Job drawing, mm, ordinate dimensions from the low corner. One solid piece. A direction names the side the tool comes from. Coordinates: 2 decimals unless noted, no trailing zeros. Loops run counter-clockwise (first coordinate to the right, second up) from the corner with the lowest first, then second, coordinate; pieces in that order, holes last. Notation, with made-up numbers: (30, 82) - (62, 82) arc R19 cw to (62, 93) - close; hole circle Ø9 at (81.25, -31.5). An arc over 180 degrees is marked (long way). Use a Markdown table: item, result. Add a question column.
1. Band-saw the part on A-A, the plane x = 11. Give the cut face in (y, z).
2. 3-axis set-ups, long thin cutter, end or side, ignore diameter. For the marked faces 4 and 5: which of +Z, -Z, +X, -X, +Y, -Y reach the whole face in a straight line?
3. Pull direction X, two halves, no side cores. Call the marked faces 1, 2 and 3: pulls with the +X half, pulls with the -X half, needs draft (parallel to the pull), parting line crosses it, or undercut.
4. Band-saw the part on D-D, the plane y = 19. Give the cut face in (x, z), plus the area to 3 significant figures.
5. Drop flat-ended pins along their axis: pin 1 (1.5 mm diameter, centred on x = 8.5, z = 2.5, fed in from +Y); pin 2 (1 mm diameter, centred on x = 3.5, z = 2, fed in from +Y); pin 3 (1.8 mm diameter, centred on x = 12.5, y = 12, fed in from +Z). Give the stop position or say it passes through.
6. Band-saw the part on C-C, the plane z = 0.5. Give the cut face in (x, y).
7. Wall check: probe 1 along Y at (x, z) = (11, 1.55); probe 2 along Y at (x, z) = (11, 2.2); probe 3 along X at (y, z) = (11.25, 0.5). Give the ranges that are in metal, low to high. Write a range as [from, to].
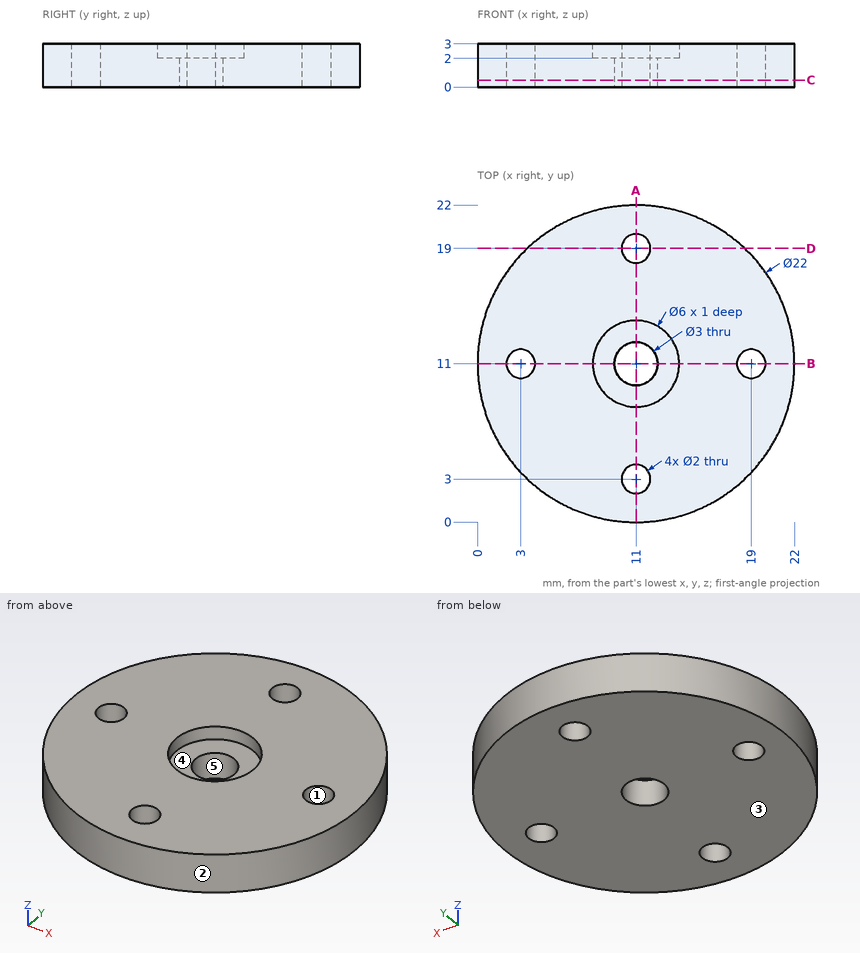
Geometry check:
| question | item | result |
|---|---|---|
| 1 | outline | (0, 0) - (2, 0) - (2, 3) - (0, 3) - close; (4, 0) - (9.5, 0) - (9.5, 2) - (8, 2) - (8, 3) - (4, 3) - close; (12.5, 0) - (18, 0) - (18, 3) - (14, 3) - (14, 2) - (12.5, 2) - close; (20, 0) - (22, 0) - (22, 3) - (20, 3) - close |
| 2 | face 4 | +Z |
| 2 | face 5 | +Z, -Z |
| 3 | face 1 | undercut |
| 3 | face 2 | parting line crosses it |
| 3 | face 3 | needs draft |
| 4 | outline | (3.45, 0) - (10, 0) - (10, 3) - (3.45, 3) - close; (12, 0) - (18.55, 0) - (18.55, 3) - (12, 3) - close |
| 4 | area | 39.3 mm^2 |
| 5 | pin 1 | stops at y = 21.86 |
| 5 | pin 2 | stops at y = 19.49 |
| 5 | pin 3 | stops at z = 2 |
| 6 | outline | circle Ø22 at (11, 11); hole circle Ø2 at (3, 11); hole circle Ø3 at (11, 11); hole circle Ø2 at (11, 3); hole circle Ø2 at (11, 19); hole circle Ø2 at (19, 11) |
| 7 | probe 1 | y = [0, 2], [4, 9.5], [12.5, 18], [20, 22] |
| 7 | probe 2 | y = [0, 2], [4, 8], [14, 18], [20, 22] |
| 7 | probe 3 | x = [0, 2.03], [3.97, 9.52], [12.48, 18.03], [19.97, 22] |
